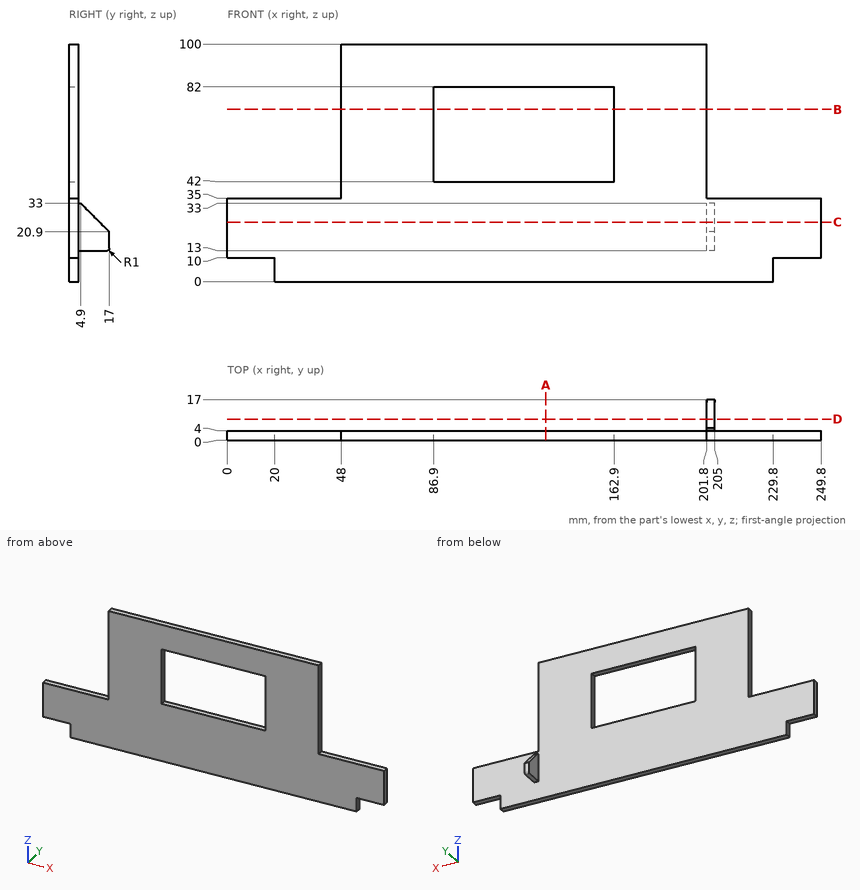
Print and shaded views of the part. All mm, measured from the part's lowest x, y and z. Coordinates: 2 decimals unless noted, no trailing zeros. Order: outer loops, then holes, each group sorted by start corner. A loop starts at its lowest first (then second) coordinate and runs counter-clockwise, first axis right, second up. Notation, with made-up numbers: (20, 60.5) -> (36, 60.5) arc R24 cw to (36, 95.5) -> close; hole circle Ø8 at (-28, -7.75). An arc over 180 degrees is marked (long way). Answer as a JSON object with one key per item and string values. Group by question number.
1) Cut at A-A, the plane x = 134. Write the cut outline in (y, z), then the cut area to 3 significant figures.
2) Cut at D-D, the plane y = 8.75. Write the cut outline in (x, z), then the cut area to 3 significant figures.
3) Drill centre lines: L1, parallel to Y at x = 146, z = 11; L2, parallel to X at y = 4.5, z = 15.5. Where is each one in solid material? Low to high.
4) Cut at B-B, the plane z = 72.5. Write the cut outline in (x, y), then the cut area to 3 significant figures.
5) Cut at C-C, the plane z = 25. Write the cut outline in (x, y), then the cut area to 3 significant figures.
6) Flat gauge pins, fed straight in: pin 1 (1.2 mm diameter, centred on y = 1, z = 4.5, fed in from -X); pin 2 (2 mm diameter, centred on x = 236, y = 2, fed in from -Z); pin 3 (5 mm diameter, centred on y = 5.5, z = 68.5, fed in from +X). Where does each tip first touch, or does it go through?
Check values:
{
 "1": {"outline": "(0, 0) -> (4, 0) -> (4, 42) -> (0, 42) -> close; (0, 82) -> (4, 82) -> (4, 100) -> (0, 100) -> close", "area": "240 mm²"},
 "2": {"outline": "(201.8, 13) -> (205, 13) -> (205, 29.15) -> (201.8, 29.15) -> close", "area": "51.7 mm²"},
 "3": {"L1": "y = 0 to 4", "L2": "x = 201.8 to 205"},
 "4": {"outline": "(48, 0) -> (86.9, 0) -> (86.9, 4) -> (48, 4) -> close; (162.9, 0) -> (201.8, 0) -> (201.8, 4) -> (162.9, 4) -> close", "area": "311 mm²"},
 "5": {"outline": "(0, 0) -> (249.8, 0) -> (249.8, 4) -> (205, 4) -> (205, 12.9) -> (201.8, 12.9) -> (201.8, 4) -> (0, 4) -> close", "area": "1,030 mm²"},
 "6": {"pin 1": "stops at x = 20", "pin 2": "stops at z = 10", "pin 3": "stops at x = 201.8"}
}
